The listing builds one solid part. Answer for the finished solid, in the listing's coordinates (mm). A direction names the side the tool comes from. Give positions to 0.01 mm unless a question says otherwise; leave off trailing zeros. Loops run counter-clockwise (first coordinate to the right, second up) from the corner with the lowest first, then second, coordinate; pieces in that order, holes last. Notation, with made-up numbers: M 48,86 L 94,86 A9 ccw 94,92 Z; hole C 26.5,-26.75 d11. An arc over 180 degrees is marked long. One line per item, written item: value. Start each with the question number.
Q1. The mould has two halves that part along X. Classify faces 1 (the flat face through (-12.2, -15, 148)), 2 (the flat face through (-2, 3, 0)), 3 (the flat face through (20, -10, 148)), 4 (the flat face through (-20, 10, 148)): +X half, -X half, draft (parallel to the pull), parting line (faces both ways), or undercut.
Q2. A cutting plane is placed at C-C, the plane z = 266. State how many separate pieces and enclosed holes the cut face has, and give its area (3 significant figures).
Q3. Flat-ended cylindrical pins translate along their axes: pin 1 (0.8 mm diameter, centred on y = -19.5, z = 119, fed in from +X); pin 2 (1.1 mm diameter, centred on x = 19.5, z = 151.5, fed in from +Y). Find the tip coordinate at first contact, or state that the pin passes through.
Q4. Consider L1, parallel to X at y = -14, z = 238; L2, parallel to Y at x = 4.5, z = 258.5. Determine where each line is inside the solid, lowest interval first.
Q5. A cutting plane is placed at A-A, the plane x = 0. Determine the outline of the cut face in (y, z), and give its area (3 significant figures).
Q6. For faces 5 (the flat face through (-7.534, -8.948, 147.9)), 6 (the flat face through (10, -20, 148)), determine the directions among +Z, -Z, +X, -X, +Y, -Y from which every point of the face is accessible in a straight line to the end or side of a thin tool.
from build123d import *

# Parameters (mm, degrees)
SKETCH3_R           = 3.4
BOSS_EXTRUDE1_DEPTH = 300


with BuildPart() as part:
    # Sketch3 → Boss-Extrude1 (new body)
    with BuildSketch(Plane.XY):
        with BuildLine():
            Line((-11.814213562, 10.4), (-6, 4.585786438))
            Line((-6, 4.585786438), (-6, -4.585786438))
            Line((-6, -4.585786438), (-11.814213562, -10.4))
            Line((-11.814213562, -10.4), (-18.2, -10.4))
            Line((-18.2, -10.4), (-18.2, -7.1))
            Line((-18.2, -7.1), (-15.5, -7.1))
            Line((-15.5, -7.1), (-15.5, -4.1))
            Line((-15.5, -4.1), (-19, -4.1))
            Line((-19, -4.1), (-19, -5.1))
            Line((-19, -5.1), (-20, -5.1))
            Line((-20, -5.1), (-20, -15.5))
            ThreePointArc((-20, -15.5), (-18.681980515, -18.681980515), (-15.5, -20))
            Line((-15.5, -20), (-5.1, -20))
            Line((-5.1, -20), (-5.1, -19))
            Line((-5.1, -19), (-4.1, -19))
            Line((-4.1, -19), (-4.1, -15.5))
            Line((-4.1, -15.5), (-7.258114106, -15.5))
            Line((-7.258114106, -15.5), (-7.258114106, -18.2))
            Line((-7.258114106, -18.2), (-10.4, -18.2))
            Line((-10.4, -18.2), (-10.4, -11.814213562))
            Line((-10.4, -11.814213562), (-4.585786438, -6))
            Line((-4.585786438, -6), (4.585786438, -6))
            Line((4.585786438, -6), (10.4, -11.814213562))
            Line((10.4, -11.814213562), (10.4, -18.2))
            Line((10.4, -18.2), (7.258114106, -18.2))
            Line((7.258114106, -18.2), (7.258114106, -15.5))
            Line((7.258114106, -15.5), (4.1, -15.5))
            Line((4.1, -15.5), (4.1, -19))
            Line((4.1, -19), (5.1, -19))
            Line((5.1, -19), (5.1, -20))
            Line((5.1, -20), (15.5, -20))
            ThreePointArc((15.5, -20), (18.681980515, -18.681980515), (20, -15.5))
            Line((20, -15.5), (20, -5.1))
            Line((20, -5.1), (19, -5.1))
            Line((19, -5.1), (19, -4.1))
            Line((19, -4.1), (15.5, -4.1))
            Line((15.5, -4.1), (15.5, -7.1))
            Line((15.5, -7.1), (18.2, -7.1))
            Line((18.2, -7.1), (18.2, -10.4))
            Line((18.2, -10.4), (11.814213562, -10.4))
            Line((11.814213562, -10.4), (6, -4.585786438))
            Line((6, -4.585786438), (6, 4.585786438))
            Line((6, 4.585786438), (11.814213562, 10.4))
            Line((11.814213562, 10.4), (18.2, 10.4))
            Line((18.2, 10.4), (18.2, 7.1))
            Line((18.2, 7.1), (15.5, 7.1))
            Line((15.5, 7.1), (15.5, 4.1))
            Line((15.5, 4.1), (19, 4.1))
            Line((19, 4.1), (19, 5.1))
            Line((19, 5.1), (20, 5.1))
            Line((20, 5.1), (20, 15.5))
            ThreePointArc((20, 15.5), (18.681980515, 18.681980515), (15.5, 20))
            Line((15.5, 20), (5.1, 20))
            Line((5.1, 20), (5.1, 19))
            Line((5.1, 19), (4.1, 19))
            Line((4.1, 19), (4.1, 15.5))
            Line((4.1, 15.5), (7.258114106, 15.5))
            Line((7.258114106, 15.5), (7.258114106, 18.2))
            Line((7.258114106, 18.2), (10.4, 18.2))
            Line((10.4, 18.2), (10.4, 11.814213562))
            Line((10.4, 11.814213562), (4.585786438, 6))
            Line((4.585786438, 6), (-4.585786438, 6))
            Line((-4.585786438, 6), (-10.4, 11.814213562))
            Line((-10.4, 11.814213562), (-10.4, 18.2))
            Line((-10.4, 18.2), (-7.258114106, 18.2))
            Line((-7.258114106, 18.2), (-7.258114106, 15.5))
            Line((-7.258114106, 15.5), (-4.1, 15.5))
            Line((-4.1, 15.5), (-4.1, 19))
            Line((-4.1, 19), (-5.1, 19))
            Line((-5.1, 19), (-5.1, 20))
            Line((-5.1, 20), (-15.5, 20))
            ThreePointArc((-15.5, 20), (-18.681980515, 18.681980515), (-20, 15.5))
            Line((-20, 15.5), (-20, 5.1))
            Line((-20, 5.1), (-19, 5.1))
            Line((-19, 5.1), (-19, 4.1))
            Line((-19, 4.1), (-15.5, 4.1))
            Line((-15.5, 4.1), (-15.5, 7.1))
            Line((-15.5, 7.1), (-18.2, 7.1))
            Line((-18.2, 7.1), (-18.2, 10.4))
            Line((-18.2, 10.4), (-11.814213562, 10.4))
        make_face()
        with BuildLine():
            Line((-18.2, -15.5), (-18.2, -12.2))
            Line((-18.2, -12.2), (-12.2, -12.2))
            Line((-12.2, -12.2), (-12.2, -18.2))
            Line((-12.2, -18.2), (-15.5, -18.2))
            ThreePointArc((-15.5, -18.2), (-17.409188309, -17.409188309), (-18.2, -15.5))
        make_face(mode=Mode.SUBTRACT)
        Circle(SKETCH3_R, mode=Mode.SUBTRACT)
        with BuildLine():
            Line((-18.2, 12.2), (-18.2, 15.5))
            ThreePointArc((-18.2, 15.5), (-17.409188309, 17.409188309), (-15.5, 18.2))
            Line((-15.5, 18.2), (-12.2, 18.2))
            Line((-12.2, 18.2), (-12.2, 12.2))
            Line((-12.2, 12.2), (-18.2, 12.2))
        make_face(mode=Mode.SUBTRACT)
        with BuildLine():
            Line((18.2, 15.5), (18.2, 12.2))
            Line((18.2, 12.2), (12.2, 12.2))
            Line((12.2, 12.2), (12.2, 18.2))
            Line((12.2, 18.2), (15.5, 18.2))
            ThreePointArc((15.5, 18.2), (17.409188309, 17.409188309), (18.2, 15.5))
        make_face(mode=Mode.SUBTRACT)
        with BuildLine():
            Line((12.2, -18.2), (12.2, -12.2))
            Line((12.2, -12.2), (18.2, -12.2))
            Line((18.2, -12.2), (18.2, -15.5))
            ThreePointArc((18.2, -15.5), (17.409188309, -17.409188309), (15.5, -18.2))
            Line((15.5, -18.2), (12.2, -18.2))
        make_face(mode=Mode.SUBTRACT)
    extrude(amount=BOSS_EXTRUDE1_DEPTH)


solid = part.part
Answer block:
1. face 1: undercut
1. face 2: draft
1. face 3: +X half
1. face 4: -X half
2. separate pieces: 1
2. enclosed holes: 5
2. area: 528 mm^2
3. pin 1: x = 18.2
3. pin 2: y = 18.39
4. L1: -20 to -18.2, -12.2 to -10.4, 10.4 to 12.2, 18.2 to 20
4. L2: -19 to -15.5, -6 to 6, 15.5 to 19
5. outline: M -6,0 L -3.4,0 L -3.4,300 L -6,300 Z; M 3.4,0 L 6,0 L 6,300 L 3.4,300 Z
5. area: 1,560 mm^2
6. face 5: +Z, -Z
6. face 6: +Z, -Z, +X, -X, -Y
